Verification items for the finished model (mm, model axes). Round coordinates to 2 decimals unless told otherwise and drop trailing zeros. Order: outer loops, then holes, each group sorted by start corner. A loop starts at its lowest first (then second) coordinate and runs counter-clockwise, first axis right, second up. Notation, with made-up numbers: M 0.25,26 L 13.25,26 A20 ccw 13.25,45 Z; hole C 38.25,61.5 d4. An arc over 180 degrees is marked long. Use one line per item in the form item = value. Start each with the question number.
Item 1: Cross-section at A-A on x = 0. Enter the section's corners in (y, z), then the cut area to 3 significant figures.
Item 2: Go/stop test with flat-tipped pins: pin 1 Ø5 at (x, z) = (55, 54.5) entering from -Y; pin 2 Ø3 at (x, y) = (48, -6.5) entering from +Z; pin 3 Ø3 at (x, z) = (46, 37.5) entering from +Y; pin 4 Ø21.5 at (x, y) = (0, 0) entering from -Z. Record where each tip stops, or that it passes through.
Item 3: Cross-section at D-D on z = 10.5. Enter the section's corners in (x, y).
Item 4: Cross-section at C-C on z = 19.5. Enter the section's corners in (x, y), then the cut area to 3 significant figures.
Item 5: Release check for a two-part mould opening along X. For faces 1 (the cylindrical face through (-15.68, -70.62, 30.98)), 2 (the cylindrical face through (16.94, 5.33, 31.01)) record: +X half, -X half, draft (parallel to the pull), parting line (faces both ways), or undercut.
Item 6: Thickness scan on probe 1 along Y at (x, z) = (0, 31.1); probe 2 along X at (y, z) = (-15, 42.5); probe 3 along Y at (x, z) = (18.5, 5). Record the ranges inside material, lowest first. Write a range as [from, to].
from build123d import *

# Parameters (mm, degrees)
F0_R     = 72.3406344385
F1_DEPTH = 61.9792044163
F2_R     = 17.7569535603
F3_DEPTH = 66.9353306293
F4_R     = 30.48


# Not quite as in the source:
# - a fillet or chamfer that OpenCascade refuses, or shapes differently, is made with other operations: its cross-section is extruded or revolved along the edge and cut away or added


with BuildPart() as f1:
    # F0 (on Top) → F1 (new body)
    with BuildSketch(Plane.XY):
        Circle(F0_R)
    extrude(amount=F1_DEPTH)

    # F2 (on face) → F3 (cut)
    with BuildSketch(Plane.XY.offset(61.9792044163)):
        Circle(F2_R)
    extrude(amount=-F3_DEPTH, mode=Mode.SUBTRACT)

    # F4
    f4_edges = [f1.edges().sort_by_distance(p)[0] for p in [
        (-72.340634, 0, 61.979204),
        (72.340634, 0, 30.989602),
        (-72.340634, 0, 0),
    ]]
    fillet(f4_edges, radius=F4_R)

    # F5: fillet of radius 30.48 on 3 edges, made by hand

    # F5_s1 → F5_t2 (revolve, cut)
    with BuildSketch(Plane.XZ):
        with BuildLine():
            ThreePointArc((41.8606344385, 61.9792044163), (24.5369471591, 51.3397369094), (17.7569535603, 32.1736184556))
            Line((17.7569535603, 32.1736184556), (17.7569535603, 61.9792044163))
            Line((17.7569535603, 61.9792044163), (41.8606344385, 61.9792044163))
        make_face()
    revolve(axis=Axis((0, 0, 61.9792044163), (0, 0, 1)), mode=Mode.SUBTRACT)

    # F5_s3 → F5_t4 (revolve, cut)
    with BuildSketch(Plane.XZ):
        with BuildLine():
            ThreePointArc((41.8606344385, 0), (24.5369471591, 10.6394675069), (17.7569535603, 29.8055859606))
            Line((17.7569535603, 29.8055859606), (17.7569535603, 0))
            Line((17.7569535603, 0), (41.8606344385, 0))
        make_face()
    revolve(axis=Axis((0, 0, 0), (0, 0, 1)), mode=Mode.SUBTRACT)


solid = f1.part
Output values:
q1.outline = M -72.34,30.48 A30.48 ccw -41.86,0 A30.48 ccw -17.76,29.81 L -17.76,32.17 A30.48 ccw -41.86,61.98 A30.48 ccw -72.34,31.5 Z; M 17.76,29.81 A30.48 ccw 41.86,0 A30.48 ccw 72.34,30.48 L 72.34,31.5 A30.48 ccw 41.86,61.98 A30.48 ccw 17.76,32.17 Z
q1.area = 5,240 mm2
q2.pin_1 = -35.05
q2.pin_2 = 61.55
q2.pin_3 = 56.33
q2.pin_4 = through
q3.outline = C 0,0 d129.76; hole C 0,0 d49.3
q4.outline = C 0,0 d140.59; hole C 0,0 d39.1
q4.area = 14,300 mm2
q5.face_1 = parting line
q5.face_2 = undercut
q6.probe_1 = [-72.34, -17.76], [17.76, 72.34]
q6.probe_2 = [-68.67, -12.55], [12.55, 68.67]
q6.probe_3 = [-55.59, -24.28], [24.28, 55.59]
